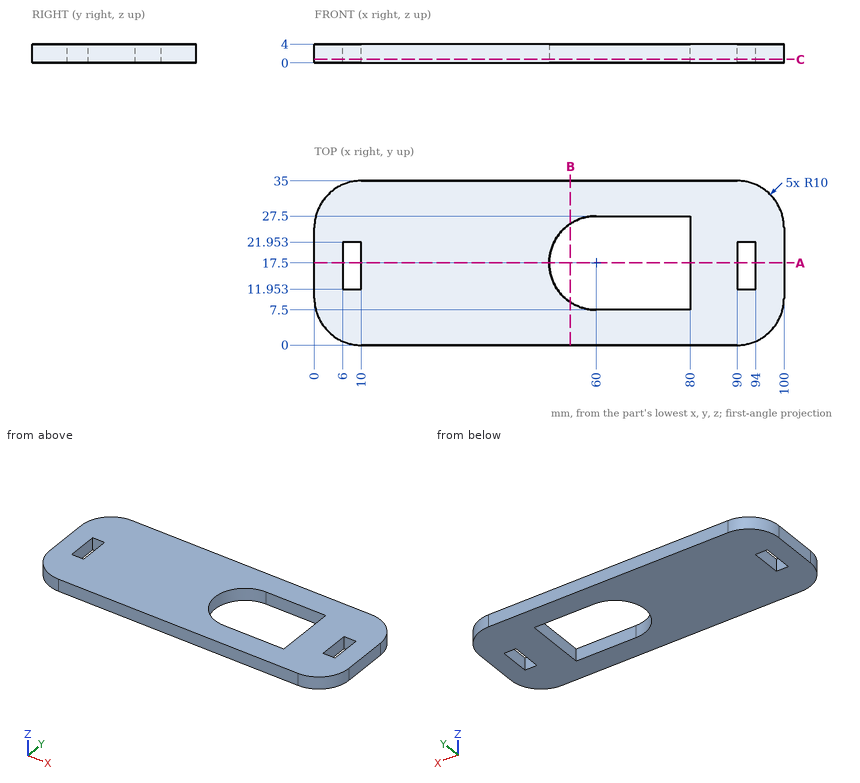
Source: three-view drawing plus pictorial views. Frame: mm from the lowest corner of the part. Round coordinates to 2 decimals unless told otherwise and drop trailing zeros. Order: outer loops, then holes, each group sorted by start corner. A loop starts at its lowest first (then second) coordinate and runs counter-clockwise, first axis right, second up. Notation, with made-up numbers: M 36.5,-24 L 40.5,-24 A12 cw 40.5,-14 Z; hole C 74,23.25 d3. An arc over 180 degrees is marked long. One line per item, written item: value.
(1) Cut plane A-A (y = 17.5). Return the cut outline in (x, z).
Result sheet:
outline: M 0,0 L 6,0 L 6,4 L 0,4 Z; M 10,0 L 50,0 L 50,4 L 10,4 Z; M 80,0 L 90,0 L 90,4 L 80,4 Z; M 94,0 L 100,0 L 100,4 L 94,4 Z
(2) Line query: probe 1 along X at (y, z) = (17.5, 1.6); probe 2 along Y at (x, z) = (71.5, 1.9); probe 3 along X at (y, z) = (15, 3.05). Output: solid intervals per line, ascending. Write a range as [from, to].
Result sheet:
probe 1: [0, 6], [10, 50], [80, 90], [94, 100]
probe 2: [0, 7.5], [27.5, 35]
probe 3: [0, 6], [10, 50.32], [80, 90], [94, 100]
(3) Pin query (flat end, axial travel): P1, Ø2, axis at y = 16, z = 2, coming from the -X side; P2, Ø1.2, axis at x = 93, z = 2, coming from the -Y side. Return the tip coordinate at first contact, or that it passes through.
Result sheet:
P1: x = 0
P2: y = 0.29
(4) Cut plane C-C (z = 0.75). Return the cut outline in (x, y), and give its area (3 significant figures).
Result sheet:
outline: M 0,10 A10 ccw 10,0 L 90,0 A10 ccw 100,10 L 100,25 A10 ccw 90,35 L 10,35 A10 ccw 0,25 Z; hole M 6,11.95 L 10,11.95 L 10,21.95 L 6,21.95 Z; hole M 60,7.5 L 80,7.5 L 80,27.5 L 60,27.5 A10 ccw Z; hole M 90,11.95 L 94,11.95 L 94,21.95 L 90,21.95 Z
area: 2,780 mm2
(5) Cut plane B-B (x = 54.5). Return the cut outline in (y, z), and give its area (3 significant figures).
Result sheet:
outline: M 0,0 L 9.15,0 L 9.15,4 L 0,4 Z; M 25.85,0 L 35,0 L 35,4 L 25.85,4 Z
area: 73.2 mm2
